Check sheet for the drawn part. Datum: minimum x, y, z corner. Units: mm. A direction names the side the tool comes from. Round coordinates to 2 decimals unless told otherwise and drop trailing zeros. Write each loop counter-clockwise with the first axis right and the second up, starting at its lowest first coordinate (ties: lowest second). Pieces come first, ordered by that corner, then holes. Notation, with made-up numbers: M -24,76.5 L -1,76.5 A28 cw -1,113.5 Z; hole C 29,47.5 d1. An arc over 180 degrees is marked long. Answer in a Markdown table with one row per item. Add a question column.
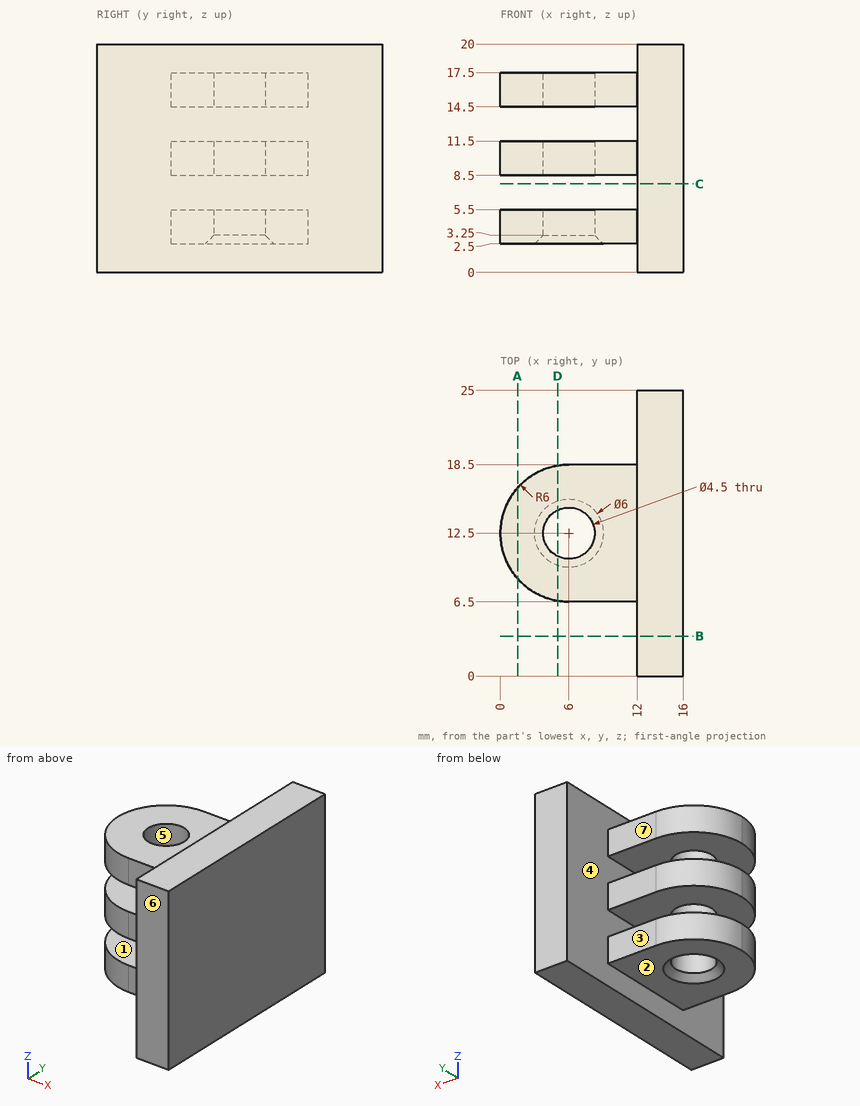
Item 1: Section check D-D, the plane x = 5. Give the number of separate pieces and of enclosed holes in the cut face, and give its area (3 significant figures).
Item 2: Section check C-C, the plane z = 7.75. Record the boundary of the cut face in (x, y), and give its area (3 significant figures).
Item 3: Access from +Z, -Z, +X, -X, +Y, -Y to the whole of each face (thin tool, end or side, straight path). Record for the marked faces 1, 2 and 3.
Item 4: Section check B-B, the plane y = 3.5. Record the boundary of the cut face in (x, z), and give its area (3 significant figures).
Item 5: Section check A-A, the plane x = 1.5. Record the boundary of the cut face in (y, z).
Item 6: Gauge pin test, flat ends, axial feed: pin 1 Ø3 at (x, z) = (10, 18) entering from +Y; pin 2 Ø7 at (x, y) = (6, 12.5) entering from +Z; pin 3 Ø1 at (y, z) = (18, 2.5) entering from -X; pin 4 Ø4 at (x, y) = (6, 12.5) entering from +Z. Record the tip position at first contact, or that the pin passes through.
Item 7: Scan lines: probe 1 along Z at (x, y) = (11.25, 17.5); probe 2 along Y at (x, z) = (6, 9.55); probe 3 along Z at (x, y) = (7.75, 14). Record each from-to range of solid material in increasing order. Write a range as from..to.
Item 8: Mould release check, pull along Y, two halves, no side actions. Record for the marked faces 4, 5, 6 and 7: +Y half, -Y half, draft (parallel to the pull), parting line (faces both ways), or undercut.
Result sheet:
| question | item | result |
|---|---|---|
| 1 | separate pieces | 6 |
| 1 | enclosed holes | 0 |
| 1 | area | 69.6 mm^2 |
| 2 | outline | M 12,0 L 16,0 L 16,25 L 12,25 Z |
| 2 | area | 100 mm^2 |
| 3 | face 1 | -X, +Y, -Y |
| 3 | face 2 | -Z, -X, +Y, -Y |
| 3 | face 3 | +Z, -Z, -X, +Y |
| 4 | outline | M 12,0 L 16,0 L 16,20 L 12,20 Z |
| 4 | area | 80.0 mm^2 |
| 5 | outline | M 8.53,2.5 L 16.47,2.5 L 16.47,5.5 L 8.53,5.5 Z; M 8.53,8.5 L 16.47,8.5 L 16.47,11.5 L 8.53,11.5 Z; M 8.53,14.5 L 16.47,14.5 L 16.47,17.5 L 8.53,17.5 Z |
| 6 | pin 1 | stops at y = 18.5 |
| 6 | pin 2 | stops at z = 17.5 |
| 6 | pin 3 | stops at x = 2.68 |
| 6 | pin 4 | passes through |
| 7 | probe 1 | z = 2.5..5.5, 8.5..11.5, 14.5..17.5 |
| 7 | probe 2 | y = 6.5..10.25, 14.75..18.5 |
| 7 | probe 3 | z = 3.2..5.5, 8.5..11.5, 14.5..17.5 |
| 8 | face 4 | draft |
| 8 | face 5 | undercut |
| 8 | face 6 | -Y half |
| 8 | face 7 | +Y half |
